Build history of the part. All positions in model axes, mm. A direction names the side the tool comes from. Round coordinates to 2 decimals unless told otherwise and drop trailing zeros. Write each loop counter-clockwise with the first axis right and the second up, starting at its lowest first coordinate (ties: lowest second). Pieces come first, ordered by that corner, then holes. Notation, with made-up numbers: (-28.75, 85.5) - (24.25, 85.5) arc R16 ccw to (24.25, 116.5) - close; hole circle Ø7 at (24, 48). An arc over 180 degrees is marked (long way). Answer as a JSON object with one key per item and string values. Group by question number.
Item 1: Slice it at B-B, the plane y = 5.1. List the corners of the cut face in (x, z), then the cut area to 3 significant figures.
Item 2: Slice it at D-D, the plane y = 0. List the corners of the cut face in (x, z).
Item 3: Flat gauge pins, fed straight in: pin 1 (1.5 mm diameter, centred on x = 22, y = 1, fed in from -Z); pin 2 (5.5 mm diameter, centred on x = 22.5, y = -0.5, fed in from +Z); pin 3 (2.5 mm diameter, centred on x = -24, y = 3, fed in from +Z). Where does each tip first touch, or does it go through?
Item 4: Probe line 1 (Y direction, x = 24.65, z = 29); line 2 (X direction, y = 5.1, z = 28.8); line 3 (Y direction, x = -24, z = 28). List the from-to ranges inside material, lowest first. Write a range as from..to.
Item 5: Which spindle directions (+Z, -Z, +X, -X, +Y, -Y) get a long thin tool onto all of the face, cutting with end or side? Do faces 1 (the flat face through (-24, 0, 30.45)), 2 (the flat face through (20.2, 0, 35)), 3 (the cylindrical face through (22.47, -4.81, 29.06)), 4 (the flat face through (-24, 0, 27.7)). Say none if no direction does.
Item 6: Slice it at C-C, the plane z = 4.5. List the corners of the cut face in (x, y).
Item 7: Slice it at A-A, the plane x = -24.65. List the corners of the cut face in (y, z), then the cut area to 4 significant figures.
Item 8: Two-plate mould, pull along Y, no slides. Class faces 5 (the flat face through (23, 0, 2.75)), 6 (the flat face through (10, 0, 37.9)), 7 (the flat face through (0, -10.1, 20)), 8 (the flat face through (23, 2.6, 5)): +Y half, -Y half, draft (parallel to the pull), parting line (faces both ways), or undercut.
Autodesk Inventor part; units mm, degrees
ref_plane "Plano de trabajo1" through (-110.1, 7.287, 0) normal (0, 0, 1) x (0, 1, 0)
ref_plane "Plano de trabajo2" through (20.2, 0, 0) normal (0, 1, 0) x (0, 0, -1)
ref_plane "Plano de trabajo3" through (0, -10.1, 0) normal (1, 0, 0) x (0, 1, 0)
ref_plane "Plano de trabajo1" through (-110.1, 7.287, 0) normal (0, 0, 1) x (0, 1, 0)
sketch "Boceto1" plane through (-110.1, 7.287, 0) normal (0, 0, 1) x (0, 1, 0)
  line L0 (-17.387, -89.9) -> (2.813, -89.9)
  line L1 (2.813, -89.9) -> (2.813, -130.3)
  line L2 (2.813, -130.3) -> (-17.387, -130.3)
  line L3 (-17.387, -130.3) -> (-17.387, -89.9)
  line L4 (-17.387, -89.9) -> (2.813, -130.3) construction
  line L5 (2.813, -89.9) -> (-17.387, -130.3) construction
  point P0 (-7.287, -110.1)
  dimension "d0" = 20.2
  dimension "d1" = 40.4
extrude "Extrusión1" add sketch "Boceto1" along normal blind 40.4
sketch "Boceto2" plane through (20.2, -10.1, 0) normal (1, 0, 0) x (0, 1, 0)
  line L0 (0, 0) -> (20.2, 0)
  line L1 (20.2, 0) -> (20.2, 40.4)
  line L2 (0, 40.4) -> (20.2, 40.4)
  line L3 (0, 0) -> (0, 40.4)
  line L4 (20.2, 0) -> (0, 0)
  line L5 (0, 0) -> (0, 27.7)
  line L6 (0, 27.7) -> (20.2, 27.7)
  line L7 (0, 27.7) -> (20.2, 27.7)
  line L8 (20.2, 27.7) -> (20.2, 30.45)
  line L9 (20.2, 30.45) -> (0, 30.45)
  line L10 (0, 30.45) -> (0, 27.7)
  point P0 (10.1, 0)
  dimension "d4" = 27.7
  dimension "d5" = 2.75
extrude "Extrusión2" add sketch "Boceto2" along normal blind 8 contours L3 L9 L1 L6
sketch "Boceto3" plane through (20.2, -10.1, 30.45) normal (0, 0, 1) x (0, 1, 0)
  line L0 (0, -8) -> (20.2, -8)
  line L1 (0, -8) -> (0, -2.25)
  line L2 (0, 0) -> (0, -8)
  line L3 (0, -2.25) -> (20.2, -2.25)
  line L4 (0, 0) -> (20.2, 0)
  line L5 (0, 0) -> (0, -8)
  line L6 (20.2, -8) -> (0, -8)
  line L7 (20.2, 0) -> (20.2, -8)
  line L8 (0, -2.25) -> (2.8, -2.25)
  line L9 (0, -2.25) -> (2.8, -2.25) construction
  line L10 (2.8, -2.25) -> (2.8, -8)
  line L11 (20.2, -8) -> (0, -8)
  circle A0 centre (5, -4.45) radius 2.2
  point P0 (10.1, 20.2)
  dimension "d8" = 5.75
  dimension "d9" = 2.8
  dimension "d10" = 0
  dimension "d11" = 90
  dimension "d12" = 4.4
hole "Agujero1" at (24.65, -5.1, 30.45) direction (0, 0, -1) diameter 4.4 end through all
ref_plane "Plano de trabajo2" through (20.2, 0, 0) normal (0, 1, 0) x (0, 0, -1)
mirror "Simetría1" about plane through (20.2, 0, 0) normal (0, 1, 0) of "Agujero1"
ref_plane "Plano de trabajo3" through (0, -10.1, 0) normal (1, 0, 0) x (0, 1, 0)
mirror "Simetría2" about plane through (0, -10.1, 0) normal (1, 0, 0) of "Extrusión2", "Agujero1", "Simetría1"
sketch "Boceto4" plane through (-110.1, 7.287, 40.4) normal (0, 0, 1) x (0, 1, 0)
  line L0 (-17.387, -130.3) -> (2.813, -130.3)
  line L1 (2.813, -130.3) -> (2.813, -89.9)
  line L2 (2.813, -89.9) -> (-17.387, -89.9)
  line L3 (-17.387, -89.9) -> (-17.387, -130.3)
  line L4 (-17.387, -130.3) -> (2.813, -130.3)
  line L5 (-7.287, -130.3) -> (-7.287, -123.6)
  line L6 (-7.287, -123.6) -> (-7.287, -117.6)
  circle A0 centre (-7.287, -120.6) radius 3
  point P0 (-7.287, -110.1)
  dimension "d20" = 6.7
  dimension "d21" = 6
extrude "Extrusión3" add sketch "Boceto4" along normal blind 4 contours A0 L6 | L6 A0
sketch "Boceto5" plane through (10.5, 0, 44.4) normal (0, 0, 1) x (1, 0, 0)
  circle A0 centre (0, 0) radius 3
  point P0 (-10.5, 0)
hole "Agujero2" at (10.5, 0, 44.4) direction (0, 0, -1) diameter 4.4 depth 6.5
sketch "Boceto6" plane through (20.2, -10.1, 0) normal (1, 0, 0) x (0, 1, 0)
  line L0 (20.2, 0) -> (20.2, 27.7)
  line L1 (0, 0) -> (20.2, 0)
  line L2 (20.2, 0) -> (20.2, 6.45)
  line L3 (20.2, 6.45) -> (0, 6.45)
  line L4 (0, 6.45) -> (0, 0)
  line L5 (0, 0) -> (20, 0)
  line L6 (20, 0) -> (20, 2.75)
  line L7 (20, 2.75) -> (0, 2.75)
  line L8 (0, 2.75) -> (0, 0)
  line L9 (0, 2.75) -> (7.5, 2.75)
  line L10 (7.5, 2.75) -> (7.5, 6.45)
  line L11 (20.2, 6.45) -> (12.7, 6.45)
  line L12 (7.5, 2.75) -> (12.7, 2.75)
  line L13 (12.7, 2.75) -> (12.7, 6.45)
  line L14 (12.7, 6.45) -> (7.5, 6.45)
  line L15 (7.5, 6.45) -> (7.5, 2.75)
  point P0 (10.1, 0)
  dimension "d31" = 6.45
  dimension "d32" = 2.75
  dimension "d33" = 7.5
  dimension "d34" = 7.5
extrude "Extrusión4" add sketch "Boceto6" along normal blind 5 contours L13 L7 L10 L3
properties part number "Servomotor"
Geometry says:
{
 "1": {"outline": "(-28.2, 27.7) - (-26.85, 27.7) - (-26.85, 30.45) - (-28.2, 30.45) - close; (-22.45, 27.7) - (-20.2, 27.7) - (-20.2, 0) - (20.2, 0) - (20.2, 27.7) - (22.45, 27.7) - (22.45, 30.45) - (20.2, 30.45) - (20.2, 40.4) - (-20.2, 40.4) - (-20.2, 30.45) - (-22.45, 30.45) - close; (26.85, 27.7) - (28.2, 27.7) - (28.2, 30.45) - (26.85, 30.45) - close", "area": "1,650 mm^2"},
 "2": {"outline": "(-28.2, 27.7) - (-20.2, 27.7) - (-20.2, 0) - (20.2, 0) - (20.2, 2.75) - (25.2, 2.75) - (25.2, 6.45) - (20.2, 6.45) - (20.2, 27.7) - (28.2, 27.7) - (28.2, 30.45) - (20.2, 30.45) - (20.2, 40.4) - (13.5, 40.4) - (13.5, 44.4) - (12.7, 44.4) - (12.7, 37.9) - (8.3, 37.9) - (8.3, 44.4) - (7.5, 44.4) - (7.5, 40.4) - (-20.2, 40.4) - (-20.2, 30.45) - (-28.2, 30.45) - close"},
 "3": {"pin 1": "stops at z = 2.75", "pin 2": "stops at z = 40.4", "pin 3": "stops at z = 30.45"},
 "4": {"line 1": "y = -10.1..-7.3, -2.9..2.9, 7.3..10.1", "line 2": "x = -28.2..-26.85, -22.45..22.45, 26.85..28.2", "line 3": "y = -10.1..-7.2, -3..3, 7.2..10.1"},
 "5": {"face 1": "+Z, -X, +Y, -Y", "face 2": "+Z, +X, +Y, -Y", "face 3": "+Z, -Z", "face 4": "-Z, -X, +Y, -Y"},
 "6": {"outline": "(-20.2, -10.1) - (20.2, -10.1) - (20.2, -2.6) - (25.2, -2.6) - (25.2, 2.6) - (20.2, 2.6) - (20.2, 10.1) - (-20.2, 10.1) - close"},
 "7": {"outline": "(-10.1, 27.7) - (-7.3, 27.7) - (-7.3, 30.45) - (-10.1, 30.45) - close; (-2.9, 27.7) - (2.9, 27.7) - (2.9, 30.45) - (-2.9, 30.45) - close; (7.3, 27.7) - (10.1, 27.7) - (10.1, 30.45) - (7.3, 30.45) - close", "area": "31.35 mm^2"},
 "8": {"face 5": "draft", "face 6": "undercut", "face 7": "-Y half", "face 8": "+Y half"}
}
